The model under review builds one solid part; all positions refer to its coordinate system, in mm. A direction names the side the tool comes from. Give positions to 0.01 mm unless a question says otherwise; leave off trailing zeros. Order: outer loops, then holes, each group sorted by start corner. A loop starts at its lowest first (then second) coordinate and runs counter-clockwise, first axis right, second up.
Autodesk Inventor part; units mm, degrees
ref_plane "YZ Plane" through (0, 0, 0) normal (1, 0, 0) x (0, 1, 0)
ref_plane "XZ Plane" through (0, 0, 0) normal (0, 1, 0) x (-1, 0, 0)
ref_plane "XY Plane" through (0, 0, 0) normal (0, 0, 1) x (1, 0, 0)
sketch "Sketch1" plane through (0, 0, 0) normal (0, 1, 0) x (-1, 0, 0)
  circle A0 centre (0, 0) radius 1.5
  dimension "d0" = 3
extrude "Extrusion1" add sketch "Sketch1" along normal blind 2
sketch "Sketch2" plane through (0, 0, 0) normal (0, -1, 0) x (1, 0, 0)
  circle A0 centre (0, 0) radius 2
  dimension "d3" = 4
extrude "Extrusion2" add sketch "Sketch2" along normal blind 4
fillet "Fillet1" radius 1 1 edges at (1.5, 2, 0)
chamfer "Chamfer1" distance 0.5 angle 45 1 edges at (-2, -4, 0)
properties part number "Circular Module"
1. To check wall thickness, follow line 1 (Z direction, x = 0.3, y = 0.75); line 2 (Y direction, x = 0.2, z = -1.35); line 3 (X direction, y = -0.5, z = 1.65). State the ranges of each line that lie inside material, in increasing order.
2. For faces 1 (the cylindrical face through (1.5, 0.49, -0.07)), 2 (the cylindrical face through (0, -2, 2)), list the 3-axis set-ups (+Z, -Z, +X, -X, +Y, -Y) from which the entire face can be reached by the end or side of a thin tool; tool diameter is ignored.
3. Take a section at A-A (y = -0.25). Write out the cut boundary in (x, z).
4. Insertion check: pin 1 (2 mm diameter, centred on x = -1.5, y = -0.5, fed in from +Z); pin 2 (1.5 mm diameter, centred on y = -2.5, z = 1, fed in from -X). Each pin has a flat end and moves straight along its axis. Give the tip position at first contact, or say it passes through.
Answer:
1. line 1: z = -1.47 to 1.47
1. line 2: y = -4 to 1.5
1. line 3: x = -1.13 to 1.13
2. face 1: +Y
2. face 2: +Y, -Y
3. outline: circle Ø4 at (0, 0)
4. pin 1: stops at z = 1.94
4. pin 2: stops at x = -1.98
